```python
from build123d import *
from build123d.topology import SkipClean

# Parameters (mm, degrees)
BOSS_EXTRUDE1_DEPTH = 3.175
SKETCH2_W           = 10.16
SKETCH2_H           = 7.62
BOSS_EXTRUDE2_DEPTH = 11.43
SKETCH3_W           = 5.08
SKETCH3_H           = 7.62
REVOLVE1_ANGLE      = 180
SKETCH4_W           = 5.08
SKETCH4_H           = 7.62
REVOLVE2_ANGLE      = 180
BOSS_EXTRUDE3_DEPTH = 15.24
SKETCH6_R           = 13.97
BOSS_EXTRUDE4_DEPTH = 3.175
FILLET1_R           = 1.27
FILLET2_R           = 0.635
BOSS_EXTRUDE5_DEPTH = 1.905
SKETCH9_R           = 1.5875
CUT_EXTRUDE1_DEPTH  = 50.746282631
CUT_EXTRUDE2_DEPTH  = 1.27
SKETCH10_R          = 1.905
BOSS_EXTRUDE6_DEPTH = 25.4
SKETCH12_R          = 13.6525
BOSS_EXTRUDE7_DEPTH = 38.1
SKETCH13_R          = 3.175
BOSS_EXTRUDE8_DEPTH = 2.54
SKETCH14_W          = 2.54
SKETCH14_H          = 0.635
BOSS_EXTRUDE9_DEPTH = 5.08
SKETCH15_R          = 0.635
CUT_EXTRUDE3_DEPTH  = 58.971361572


with BuildPart() as part:
    # Sketch1 → Boss-Extrude1 (new body)
    with BuildSketch(Plane.XY):
        Polygon((-19.3675, 27.94), (-19.3675, 0), (19.3675, 0), (19.3675, 27.94), (8.255, 38.735), (-8.255, 38.735), align=None)
    extrude(amount=BOSS_EXTRUDE1_DEPTH)

    # Sketch2 → Boss-Extrude2 (add)
    with BuildSketch(Plane.XY.offset(3.175)):
        with Locations((-8.255, 3.81)):
            Rectangle(SKETCH2_W, SKETCH2_H)
        with Locations((8.255, 3.81)):
            Rectangle(SKETCH2_W, SKETCH2_H)
    extrude(amount=BOSS_EXTRUDE2_DEPTH)

    # Sketch3 → Revolve1 (revolve)
    with SkipClean():  # the faces are left unmerged after this step: merging them gives an invalid solid
        with BuildSketch(Plane.XY.offset(14.605)):
            with Locations((-5.715, 3.81)):
                Rectangle(SKETCH3_W, SKETCH3_H)
            with Locations((-10.795, 3.81)):
                Rectangle(SKETCH3_W, SKETCH3_H)
        revolve(axis=Axis((-8.255, 7.62, 14.605), (0, -1, 0)), revolution_arc=REVOLVE1_ANGLE)
    add(part.part.scale(1), mode=Mode.REPLACE)  # the faces are merged on a copy

    # Sketch4 → Revolve2 (revolve)
    with BuildSketch(Plane.XY.offset(14.605)):
        with Locations((5.715, 3.81)):
            Rectangle(SKETCH4_W, SKETCH4_H)
    revolve(axis=Axis((8.255, 7.62, 14.605), (0, 1, 0)), revolution_arc=REVOLVE2_ANGLE)

    # Sketch5 → Boss-Extrude3 (add)
    with BuildSketch(Plane.XY.offset(3.175)):
        with BuildLine():
            ThreePointArc((14.352662754, 12.90143922), (0, 35.56), (-14.352662754, 12.90143922))
            Line((-14.352662754, 12.90143922), (-11.856473401, 7.62))
            Line((-11.856473401, 7.62), (-3.175, 7.62))
            Line((-3.175, 7.62), (-3.175, 3.81))
            Line((-3.175, 3.81), (3.175, 3.81))
            Line((3.175, 3.81), (3.175, 7.62))
            Line((3.175, 7.62), (11.856473401, 7.62))
            Line((11.856473401, 7.62), (14.352662754, 12.90143922))
        make_face()
    extrude(amount=BOSS_EXTRUDE3_DEPTH)

    # Sketch6 → Boss-Extrude4 (add)
    with BuildSketch(Plane.XY.offset(18.415)):
        with Locations(Location((0, 19.685, 0), (0, 0, 239.727358681))):
            Circle(SKETCH6_R)
    extrude(amount=BOSS_EXTRUDE4_DEPTH)

    # Fillet1
    fillet1_edges = [part.edges().sort_by_distance(p)[0] for p in [
        (7.042490682, 31.75, 21.59),
    ]]
    fillet(fillet1_edges, radius=FILLET1_R)

    # Fillet2
    # the kernel refuses this fillet: 0.635 mm, written as the material it takes off along each edge
    with BuildSketch(Plane(origin=(11.178117323, 6.184733725, 18.415), x_dir=(-0.9041047404261693, 0.4273109153051544, 0), z_dir=(0.42731091530515436, 0.9041047404261694, 0))) as fillet2_piece_1_section:
        with BuildLine():
            CenterArc((FILLET2_R, -FILLET2_R), FILLET2_R, 90, 90)
            Line((0, -FILLET2_R), (0, 0))
            Line((0, 0), (FILLET2_R, 0))
        make_face()
    fillet2_piece_1 = extrude(amount=7.429123192, mode=Mode.PRIVATE)
    fillet2_piece_1 = split(fillet2_piece_1, bisect_by=Plane(origin=(12.958569615, 7.62, 18.272124555), z_dir=(0, 1, 0)), keep=Keep.TOP, mode=Mode.PRIVATE)
    add(fillet2_piece_1, mode=Mode.SUBTRACT)
    with BuildSketch(Plane(origin=(0, 19.685, 18.415), x_dir=(0.9041047404261693, -0.42731091530515447, 0), z_dir=(-0.42731091530515447, -0.9041047404261693, 0))) as fillet2_piece_2:
        with BuildLine():
            CenterArc((15.875 - FILLET2_R, -FILLET2_R), FILLET2_R, 0, 90)
            Line((15.875, -FILLET2_R), (15.875, 0))
            Line((15.875, 0), (15.875 - FILLET2_R, 0))
        make_face()
    revolve(axis=Axis((0, 19.685, 18.415), (0, 0, 1)), revolution_arc=230.594049451, mode=Mode.SUBTRACT)
    with BuildSketch(Plane(origin=(-14.352662754, 12.90143922, 18.415), x_dir=(0.9041047404261693, 0.4273109153051546, 0), z_dir=(0.4273109153051546, -0.9041047404261694, 0))) as fillet2_piece_3_section:
        with BuildLine():
            CenterArc((FILLET2_R, -FILLET2_R), FILLET2_R, 90, 90)
            Line((0, -FILLET2_R), (0, 0))
            Line((0, 0), (FILLET2_R, 0))
        make_face()
    fillet2_piece_3 = extrude(amount=7.429123192, mode=Mode.PRIVATE)
    fillet2_piece_3 = split(fillet2_piece_3, bisect_by=Plane(origin=(-12.958569615, 7.62, 18.272124555), z_dir=(0, 1, 0)), keep=Keep.TOP, mode=Mode.PRIVATE)
    add(fillet2_piece_3, mode=Mode.SUBTRACT)

    # Sketch8 → Boss-Extrude5 (add)
    with BuildSketch(Plane.XZ):
        Polygon((-22.5425, 0), (-22.5425, -10.795), (-14.2875, -10.795), (-6.985, 0), align=None)
        Polygon((22.5425, -10.795), (14.2875, -10.795), (6.985, 0), (22.5425, 0), align=None)
    extrude(amount=-BOSS_EXTRUDE5_DEPTH)

    # Sketch9 → Cut-Extrude1 (cut, through all)
    with BuildSketch(Plane.XZ):
        with Locations(Location((18.415, -4.7625, 0), (0, 0, 270))):
            Circle(SKETCH9_R)
        with Locations(Location((-18.415, -4.7625, 0), (0, 0, 270))):
            Circle(SKETCH9_R)
    extrude(amount=-CUT_EXTRUDE1_DEPTH, mode=Mode.SUBTRACT)

    # Sketch11 → Cut-Extrude2 (cut)
    with BuildSketch(Plane.XZ):
        with BuildLine():
            Line((-11.43, 6.985), (-5.08, 6.985))
            Line((-5.08, 6.985), (-5.08, 14.605))
            ThreePointArc((-5.08, 14.605), (-8.255, 17.78), (-11.43, 14.605))
            Line((-11.43, 14.605), (-11.43, 6.985))
        make_face()
        with BuildLine():
            Line((11.43, 14.605), (11.43, 6.985))
            Line((11.43, 6.985), (5.08, 6.985))
            Line((5.08, 6.985), (5.08, 14.605))
            ThreePointArc((5.08, 14.605), (8.255, 17.78), (11.43, 14.605))
        make_face()
    extrude(amount=-CUT_EXTRUDE2_DEPTH, mode=Mode.SUBTRACT)

    # Sketch10 → Boss-Extrude6 (add)
    with BuildSketch(Plane.XZ.offset(-1.27)):
        with Locations(Location((-8.255, 15.24, 0), (0, 0, 270))):
            Circle(SKETCH10_R)
        with Locations(Location((8.255, 15.24, 0), (0, 0, 90))):
            Circle(SKETCH10_R)
    extrude(amount=BOSS_EXTRUDE6_DEPTH)

    # Sketch12 → Boss-Extrude7 (add)
    with BuildSketch(Plane(origin=(0, 0, 0), x_dir=(-1, 0, 0), z_dir=(0, 0, -1))):
        with Locations(Location((0, 19.685, 0), (0, 0, 180))):
            Circle(SKETCH12_R)
    extrude(amount=BOSS_EXTRUDE7_DEPTH)

    # Sketch13 → Boss-Extrude8 (add)
    with BuildSketch(Plane(origin=(0, 0, -38.1), x_dir=(-1, 0, 0), z_dir=(0, 0, -1))):
        with Locations((0, 19.685)):
            Circle(SKETCH13_R)
    extrude(amount=BOSS_EXTRUDE8_DEPTH)

    # Sketch14 → Boss-Extrude9 (add)
    with BuildSketch(Plane(origin=(0, 0, -38.1), x_dir=(-1, 0, 0), z_dir=(0, 0, -1))):
        with Locations((0, 31.75)):
            Rectangle(SKETCH14_W, SKETCH14_H)
        with Locations((0, 7.62)):
            Rectangle(SKETCH14_W, SKETCH14_H)
    extrude(amount=BOSS_EXTRUDE9_DEPTH)

    # Sketch15 → Cut-Extrude3 (cut, through all)
    with BuildSketch(Plane.XZ.offset(-7.3025)):
        with Locations((0, -41.96981375)):
            Circle(SKETCH15_R)
    extrude(amount=-CUT_EXTRUDE3_DEPTH, mode=Mode.SUBTRACT)


solid = part.part
```
Here's how the part is built. I have some questions about the finished solid (model axes, mm). A direction names the side the tool comes from. Give positions to 0.01 mm unless a question says otherwise; leave off trailing zeros. Write each loop counter-clockwise with the first axis right and the second up, starting at its lowest first coordinate (ties: lowest second). Pieces come first, ordered by that corner, then holes. Notation, with made-up numbers: M -8,73.5 L 23,73.5 A17 ccw 23,105.5 Z; hole C 61,73 d6. An arc over 180 degrees is marked long. Put each result on its own line as item: value. Start each with the question number.
Item 1: If we section it at B-B, the plane y = -4: Write out the boundary of the cut face in (x, z) (3 decimals), then the cut area to 3 significant figures.
Item 2: Thinking about a two-plate mould opening in Z: for faces 1 (the flat face through (13.335, 4, 9)), 2 (the flat face through (-10.687, 0.939, -5.473)), 3 (the flat face through (3.8, 7.62, 17.5)), which applies, +Z half, -Z half, draft (parallel to the pull), parting line (faces both ways), or undercut?
Item 3: If we section it at A-A, the plane z = 12: Write out the boundary of the cut face in (x, y) (3 decimals), then the cut area to 3 significant figures.
Item 4: I need wall thicknesses on L1, parallel to X at y = 3, z = 13 (3 decimals); L2, parallel to Y at x = -15, z = -8 (3 decimals); L3, parallel to Y at x = 0, z = -25.5. Which ranges of each line are inside material? Lowest first, please. Write a range as from..to.
Item 5: On a 3-axis mill with a long thin cutter (end or side, diameter ignored), from which of +Z, -Z, +X, -X, +Y, -Y can I reach the whole of each face in a straight line? I mean faces 4 (the flat face through (-13.335, 4, 9)), 5 (the flat face through (-3.175, 2, 9)), 6 (the flat face through (0, 31.432, -41)), 7 (the cylindrical face through (-8.19, 0.63, 17.78)). Say none if no direction works.
Item 6: If we section it at D-D, the plane z = -13: Write out the boundary of the cut face in (x, y) (1 decimal).
Item 7: Will these pins go through, and if not, where does the flat tip stop? pin 1 (1 mm diameter, centred on x = 5, z = -21, fed in from -Y); pin 2 (0.5 mm diameter, centred on x = 4.5, z = 16, fed in from -Y); pin 3 (3 mm diameter, centred on x = -5.5, z = -20, fed in from +Y).
Item 8: If we section it at C-C, the plane z = 2: Write out the boundary of the cut face in (x, y) (1 decimal).
Values:
1. outline: C -8.255,15.24 d3.81; C 8.255,15.24 d3.81
1. area: 22.8 mm²
2. face 1: draft
2. face 2: -Z half
2. face 3: undercut
3. outline: M -14.353,12.901 L -11.856,7.62 L -13.335,7.62 L -13.335,0 L -11.43,0 L -11.43,1.27 L -5.08,1.27 L -5.08,0 L -3.175,0 L -3.175,3.81 L 3.175,3.81 L 3.175,0 L 5.08,0 L 5.08,1.27 L 11.43,1.27 L 11.43,0 L 13.335,0 L 13.335,7.62 L 11.856,7.62 L 14.353,12.901 A15.875 ccw long Z
3. area: 906 mm²
4. L1: -13.335..-3.175, 3.175..13.335
4. L2: 0..1.905
4. L3: 6.03..33.34
5. face 4: +Z, -X, -Y
5. face 5: +Z, -Y
5. face 6: -Z, +X, -X
5. face 7: -Y
6. outline: C 0,19.7 d27.3
7. pin 1: y = 6.8
7. pin 2: y = 0
7. pin 3: y = 32.74
8. outline: M -19.4,0 L 19.4,0 L 19.4,27.9 L 8.3,38.7 L -8.3,38.7 L -19.4,27.9 Z
